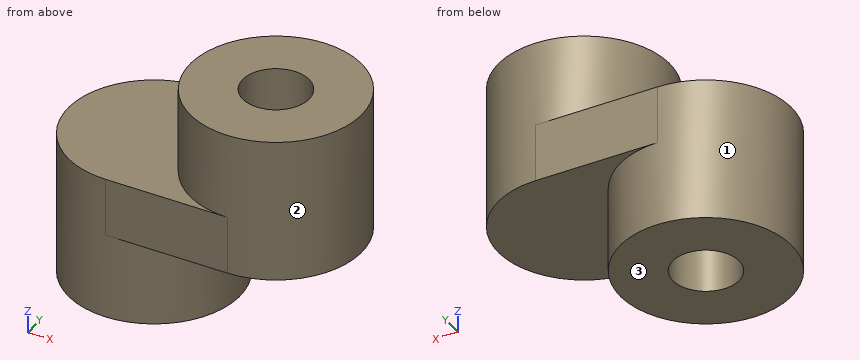
Autodesk Inventor part; units mm, degrees
ref_plane "YZ Plane" through (0, 0, 0) normal (1, 0, 0) x (0, 1, 0)
ref_plane "XZ Plane" through (0, 0, 0) normal (0, 1, 0) x (-1, 0, 0)
ref_plane "XY Plane" through (0, 0, 0) normal (0, 0, 1) x (1, 0, 0)
sketch "Sketch2" plane through (0, 0, 0) normal (0, 0, 1) x (1, 0, 0)
  arc A0 (4.563, -3.175) -> (4.563, 3.175) centre (4.563, 0) ccw
  arc A1 (0, 3.175) -> (0, -3.175) centre (0, 0) ccw
  line L0 (0, 3.175) -> (4.563, 3.175)
  line L1 (0, -3.175) -> (4.563, -3.175)
  dimension "d14" = 6.35
  dimension "d15" = 6.35
  dimension "d16" = 0
  dimension "d17" = 0
  dimension "d18" = 4.563
  dimension "d19" = 0
extrude "Extrusion2" add sketch "Sketch2" along normal blind 8.509
sketch "Sketch3" plane through (0, 0, 8.509) normal (0, 0, 1) x (1, 0, 0)
  point P0 (0, 0)
  point P1 (4.563, 0)
  dimension "d22" = 4.563
  dimension "d23" = 0
hole "Hole1" at (4.563, 0, 8.509) direction (0, 0, -1) diameter 2.459 depth 3.81 tip angle 118
sketch "Sketch4" plane through (0, 0, 0) normal (0, 0, -1) x (-1, 0, 0)
  point P0 (0, 0)
hole "Hole2" at (0, 0, 0) direction (0, 0, 1) diameter 2.459 depth 3.81 tip angle 118
sketch "Sketch7" plane through (0, 0, 0) normal (0, 0, -1) x (-1, 0, 0)
  arc A0 (0, 3.175) -> (0, -3.175) centre (0, 0) ccw
  arc A1 (-4.563, 3.175) -> (-4.563, -3.175) centre (-4.563, 0) ccw
  arc A2 (-4.563, 3.175) -> (-4.563, -3.175) centre (-4.563, 0) ccw
  line L0 (0, -3.175) -> (-4.563, -3.175)
  line L1 (-4.563, -3.175) -> (0, -3.175)
  line L2 (0, 3.175) -> (-4.563, 3.175)
extrude "Extrusion5" cut sketch "Sketch7" against normal blind 3.175
sketch "Sketch8" plane through (0, 0, 8.509) normal (0, 0, 1) x (1, 0, 0)
  arc A0 (0, 3.175) -> (0, -3.175) centre (0, 0) ccw
  arc A1 (4.563, 3.175) -> (4.563, -3.175) centre (4.563, 0) ccw
  line L0 (4.563, 3.175) -> (0, 3.175)
  line L1 (0, 3.175) -> (4.563, 3.175)
  line L2 (0, -3.175) -> (4.563, -3.175)
  line L3 (4.563, -3.175) -> (0, -3.175)
sketch "Sketch8 outline for Extrusion6" plane through (0, 0, 8.509) normal (0, 0, 1) x (1, 0, 0)
  arc A0 (0, 3.175) -> (0, -3.175) centre (0, 0) ccw
  line L0 (4.563, 3.175) -> (0, 3.175)
  arc A1 (4.563, -3.175) -> (4.563, 3.175) centre (4.563, 0) cw
  line L1 (0, -3.175) -> (4.563, -3.175)
extrude "Extrusion6" cut sketch "Sketch8 outline for Extrusion6" against normal blind 3.175
properties part number "PC104_EM-113 standoff_4.563"
CAD build for the part. Positions are in the model's coordinates, mm. Face numbers are marked on the shaded views. A direction names the side the tool comes from. Coordinates: 2 decimals unless noted, no trailing zeros. Loops run counter-clockwise (first coordinate to the right, second up) from the corner with the lowest first, then second, coordinate; pieces in that order, holes last. Notation, with made-up numbers: (46, 33.5) - (60, 33.5) arc R16 cw to (60, 38.5) - close; hole circle Ø11 at (1, 46.5). An arc over 180 degrees is marked (long way). Return JSON: item names as keys, results as strings.
1. Band-saw the part on D-D (x = -1.5). Give the cut face in (y, z).
Result:
{"outline": "(-2.8, 0) - (2.8, 0) - (2.8, 5.33) - (-2.8, 5.33) - close"}
2. 3-axis set-ups, long thin cutter, end or side, ignore diameter. For the marked faces 1, 2 and 3: which of +Z, -Z, +X, -X, +Y, -Y reach the whole face in a straight line?
Result:
{"face 1": "-Z", "face 2": "+Z", "face 3": "-Z, +X, -X, +Y, -Y"}
3. Probe L1, parallel to X at y = 0, z = 6.45; L2, parallel to X at y = 0, z = 1.3 (1 decimal). List the from-to ranges inside material, lowest first. Write a range as from..to.
Result:
{"L1": "x = 1.39..3.33, 5.79..7.74", "L2": "x = -3.2..-1.2, 1.2..3.2"}
4. Drop flat-ended pins along their axis: pin 1 (2 mm diameter, centred on y = -1.5, z = 7, fed in from -X); pin 2 (2 mm diameter, centred on x = 4.563, y = 0, fed in from -Z) (3 decimals); pin 3 (2 mm diameter, centred on x = 0, y = 0, fed in from -Z). Give the stop position or say it passes through.
Result:
{"pin 1": "stops at x = 1.43", "pin 2": "stops at z = 3.175", "pin 3": "stops at z = 3.95"}
5. Band-saw the part on B-B (y = -2.5). Give the cut face in (x, z) (3 decimals).
Result:
{"outline": "(-1.957, 0) - (1.957, 0) - (1.957, 3.175) - (6.52, 3.175) - (6.52, 8.509) - (2.606, 8.509) - (2.606, 5.334) - (-1.957, 5.334) - close"}
